```python
from build123d import *

# Parameters (mm, degrees)
F0_W     = 152.4
F0_H     = 114.3
F1_DEPTH = 12.7
F2_DEPTH = 50.8


with BuildPart() as f1:
    # F0 (on Top) → F1 (new body)
    with BuildSketch(Plane.XY):
        with Locations((0, 0.099638)):
            Rectangle(F0_W, F0_H)
        with BuildLine():
            Line((-28.260375, -10.299862), (-8.980256, 8.980256))
            Line((-8.980256, 8.980256), (11.128381, 29.088893))
            ThreePointArc((11.128381, 29.088893), (29.213265, 29.088893), (29.213265, 11.004009))
            Line((29.213265, 11.004009), (9.104628, -9.104628))
            Line((9.104628, -9.104628), (-10.175491, -28.384746))
            ThreePointArc((-10.175491, -28.384746), (-28.260375, -28.384746), (-28.260375, -10.299862))
        make_face(mode=Mode.SUBTRACT)
        with BuildLine():
            Line((11.128381, 29.088893), (-8.980256, 8.980256))
            Line((-8.980256, 8.980256), (-28.260375, -10.299862))
            ThreePointArc((-28.260375, -10.299862), (-28.260375, -28.384746), (-10.175491, -28.384746))
            Line((-10.175491, -28.384746), (9.104628, -9.104628))
            Line((9.104628, -9.104628), (29.213265, 11.004009))
            ThreePointArc((29.213265, 11.004009), (29.213265, 29.088893), (11.128381, 29.088893))
        make_face()
    extrude(amount=F1_DEPTH)

    # F0 (on Top) → F2 (join)
    with BuildSketch(Plane.XY):
        with BuildLine():
            Line((11.128381, 29.088893), (-8.980256, 8.980256))
            Line((-8.980256, 8.980256), (-28.260375, -10.299862))
            ThreePointArc((-28.260375, -10.299862), (-28.260375, -28.384746), (-10.175491, -28.384746))
            Line((-10.175491, -28.384746), (9.104628, -9.104628))
            Line((9.104628, -9.104628), (29.213265, 11.004009))
            ThreePointArc((29.213265, 11.004009), (29.213265, 29.088893), (11.128381, 29.088893))
        make_face()
    extrude(amount=F2_DEPTH)


solid = f1.part
```
Geometry: final body of the model. Coordinates: model frame, mm. A direction names the side the tool comes from. Coordinates: 2 decimals unless noted, no trailing zeros. Order: outer loops, then holes, each group sorted by start corner. A loop starts at its lowest first (then second) coordinate and runs counter-clockwise, first axis right, second up. Notation, with made-up numbers: (74.5, 30) - (123.5, 30) arc R23 ccw to (123.5, 65) - close; hole circle Ø10 at (26, 77.25). An arc over 180 degrees is marked (long way). Write each question's results on one line, items separated by ' | '.
1) Set-up query: faces 1 (the flat face through (-18, 1, 12.7)), 2 (the flat face through (-76.2, -1, 6)). Return all of +Z, -Z, +X, -X, +Y, -Y with unobstructed straight access to the full face (end or side cutting, diameter ignored); none if empty.
Results list:
face 1: +Z | face 2: +Z, -Z, -X, +Y, -Y
2) Pull-direction query (X, two-part tool) for faces 3 (the flat face through (76.2, -1, 6)), 4 (the cylindrical face through (29.4, 28.9, 31.5)), 5 (the flat face through (-1, -57.05, 6)); classes: pulls with the +X half, pulls with the -X half, needs draft (parallel to the pull), parting line crosses it, or undercut.
Results list:
face 3: pulls with the +X half | face 4: parting line crosses it | face 5: needs draft
3) Line query: line 1 (Z direction, x = -56, y = 21); line 2 (X direction, y = 10, z = 16.5); line 3 (X direction, y = -10.5, z = 18). Output: solid intervals per line, ascending. Write a range as from..to.
Results list:
line 1: 0..12.7 | line 2: -7.96..28.21 | line 3: -28.46..7.71
4) Section C-C, the plane y = 15.5. Return loops of the section in (x, z), plus the area to 3 significant figures.
Results list:
outline: (-76.2, 0) - (76.2, 0) - (76.2, 12.7) - (32.12, 12.7) - (32.12, 50.8) - (-2.46, 50.8) - (-2.46, 12.7) - (-76.2, 12.7) - close | area: 3,250 mm^2
5) Pin query (flat end, axial travel): pin 1 (6 mm diameter, centred on x = -28.5, z = 34, fed in from -Y); pin 2 (8 mm diameter, centred on x = -32, z = 22, fed in from -Y); pin 3 (1.5 mm diameter, centred on y = -16, z = 35.5, fed in from +X). Return the tip coordinate at first contact, or that it passes through.
Results list:
pin 1: y = -30.48 | pin 2: y = -28.64 | pin 3: x = 2.96
6) Section B-B, the plane x = 2. Return loops of the section in (y, z), plus the area to 3 significant figures.
Results list:
outline: (-57.05, 0) - (57.25, 0) - (57.25, 12.7) - (19.96, 12.7) - (19.96, 50.8) - (-16.21, 50.8) - (-16.21, 12.7) - (-57.05, 12.7) - close | area: 2,830 mm^2
7) Section D-D, the plane y = -49. Return loops of the section in (x, z).
Results list:
outline: (-76.2, 0) - (76.2, 0) - (76.2, 12.7) - (-76.2, 12.7) - close
